For this review, take the finished solid that the model builds, in its own axes (mm). Coordinates: 2 decimals unless noted, no trailing zeros. Write each loop counter-clockwise with the first axis right and the second up, starting at its lowest first coordinate (ties: lowest second). Pieces come first, ordered by that corner, then holes. Notation, with made-up numbers: M -20,-13.75 L -16,-13.75 A11 ccw -16,-7.75 Z; hole C 43,-4 d8. An arc over 180 degrees is marked long. One line per question, with ' | ' between items.
from build123d import *

# Parameters (mm, degrees)
SKETCH_2_W          = 35
SKETCH_2_H          = 58
EXTRUDE_1_DEPTH     = 2.5
SKETCH_4_W          = 7.5
SKETCH_4_H          = 3
CUT_EXTRUDE_1_DEPTH = 3.5
CUT_EXTRUDE_2_DEPTH = 3.5
SKETCH_7_W          = 10
SKETCH_7_H          = 10
CUT_EXTRUDE_3_DEPTH = 3.5
FILLET_1_R          = 1


with BuildPart() as part:
    # 草图2 → 凸台-拉伸1 (new body)
    with BuildSketch(Plane(origin=(0, 0, 0), x_dir=(0, 0, -1), z_dir=(1, 0, 0))):
        Rectangle(SKETCH_2_W, SKETCH_2_H)
    extrude(amount=EXTRUDE_1_DEPTH)

    # 草图4 → 切除-拉伸1 (cut, through all)
    with BuildSketch(Plane.ZY):
        with Locations((-8.95, 24.5)):
            Rectangle(SKETCH_4_W, SKETCH_4_H)
        with Locations((10.95, 24.5)):
            Rectangle(SKETCH_4_W, SKETCH_4_H)
        with Locations((-8.95, -24.5)):
            Rectangle(SKETCH_4_W, SKETCH_4_H)
        with Locations((10.95, -24.5)):
            Rectangle(SKETCH_4_W, SKETCH_4_H)
    extrude(amount=-CUT_EXTRUDE_1_DEPTH, mode=Mode.SUBTRACT)

    # 草图5 → 切除-拉伸2 (cut, through all)
    with BuildSketch(Plane.ZY):
        with BuildLine():
            Line((-17.5, 29), (-17.5, 26.000000007))
            ThreePointArc((-17.5, 26.000000007), (-16.621320341, 28.121320346), (-14.5, 29))
            Line((-14.5, 29), (-17.5, 29))
        make_face()
        with BuildLine():
            Line((-14.5, 0), (-14.5, 23))
            ThreePointArc((-14.5, 23), (-16.621320346, 23.878679659), (-17.5, 26.000000007))
            Line((-17.5, 26.000000007), (-17.5, 0))
            Line((-17.5, 0), (-14.5, 0))
        make_face()
        with BuildLine():
            Line((-14.5, -23), (-14.5, 0))
            Line((-14.5, 0), (-17.5, 0))
            Line((-17.5, 0), (-17.5, -26))
            ThreePointArc((-17.5, -26), (-16.621320344, -23.878679656), (-14.5, -23))
        make_face()
        with BuildLine():
            ThreePointArc((-14.5, -29), (-16.621320344, -28.121320344), (-17.5, -26))
            Line((-17.5, -26), (-17.5, -29))
            Line((-17.5, -29), (-14.5, -29))
        make_face()
    extrude(amount=-CUT_EXTRUDE_2_DEPTH, mode=Mode.SUBTRACT)

    # 草图7 → 切除-拉伸3 (cut, through all)
    with BuildSketch(Plane.ZY):
        with Locations((1, -11)):
            Rectangle(SKETCH_7_W, SKETCH_7_H)
        with Locations((1, 11)):
            Rectangle(SKETCH_7_W, SKETCH_7_H)
    extrude(amount=-CUT_EXTRUDE_3_DEPTH, mode=Mode.SUBTRACT)

    # 圆角1
    fillet_1_edges = [part.edges().sort_by_distance(p)[0] for p in [
        (1.25, -29, 17.5),
        (1.25, 29, 17.5),
    ]]
    fillet(fillet_1_edges, radius=FILLET_1_R)


solid = part.part
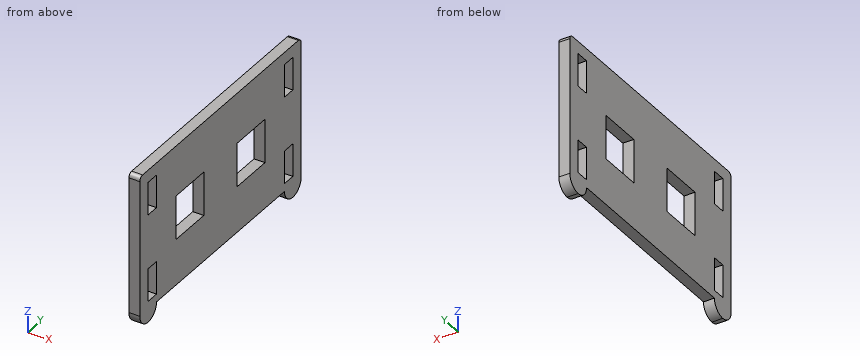
1. For line 1 along Y through (x, z) = (1.5, 10); line 2 along Z through (x, y) = (1.85, -24); line 3 along Y through (x, z) = (0.75, -3), list the stretches that pass through material, from the lowest coordinate up.
Computed values:
line 1: y = -29 to -26, -23 to 23, 26 to 29 | line 2: z = -16.74 to -12.7, -5.2 to 7.2, 14.7 to 17.5 | line 3: y = -29 to -16, -6 to 6, 16 to 29
2. Take a section at C-C on x = 1.55. Give the number of separate pieces and of enclosed holes in the cut face, plus the area to 3 significant figures.
Computed values:
separate pieces: 1 | enclosed holes: 6 | area: 1,590 mm2
3. Take a section at D-D on y = 24. State the section outline as (x, z) points.
Computed values:
outline: M 0,-16.74 L 2.5,-16.74 L 2.5,-12.7 L 0,-12.7 Z; M 0,-5.2 L 2.5,-5.2 L 2.5,7.2 L 0,7.2 Z; M 0,14.7 L 2.5,14.7 L 2.5,17.5 L 0,17.5 Z
4. Clearance check with a flat-ended pin moving along its axis: P1, Ø0.8, axis at x = 1, y = -11.5, coming from the -Z side. State where the tip first meets the part, or that it passes through.
Computed values:
P1: stops at z = -14.5
5. Take a section at A-A on z = -9. State the section outline as (x, y) points.
Computed values:
outline: M 0,-29 L 2.5,-29 L 2.5,-26 L 0,-26 Z; M 0,-23 L 2.5,-23 L 2.5,23 L 0,23 Z; M 0,26 L 2.5,26 L 2.5,29 L 0,29 Z
6. Take a section at B-B on y = -12. State the section outline as (x, z) points, plus the area to 3 significant figures.
Computed values:
outline: M 0,-14.5 L 2.5,-14.5 L 2.5,-4 L 0,-4 Z; M 0,6 L 2.5,6 L 2.5,17.5 L 0,17.5 Z | area: 55.0 mm2
